Could you check a few things on this model? Use its own coordinates, in mm. Face numbers are marked on the shaded views. A direction names the side the tool comes from. Round coordinates to 2 decimals unless told otherwise and drop trailing zeros. Loops run counter-clockwise (first coordinate to the right, second up) from the corner with the lowest first, then second, coordinate; pieces in that order, holes last. Notation, with made-up numbers: M -2.5,-24.75 L 32.5,-24.75 A27 cw 32.5,-2.75 Z; hole C 21,59.5 d10. An arc over 180 degrees is marked long. Answer in a Markdown table with one row per item.
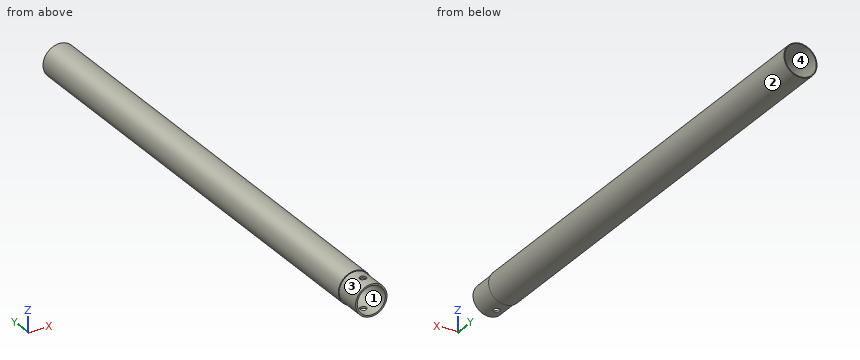
```python
from build123d import *

# Parameters (mm, degrees)
SKETCH1_R                = 31.75
SKETCH1_R_2              = 30.1625
BOSS_EXTRUDE1_DEPTH      = 914.4
BOSS_EXTRUDE2_DEPTH      = 50.8
BOSS_EXTRUDE2_DEPTH_BACK = 25.4
SKETCH3_R                = 30.1625
SKETCH3_R_2              = 26.9875
CUT_EXTRUDE2_DEPTH       = 916.501766792
CUT_EXTRUDE2_DEPTH_BACK  = 916.501766792
SKETCH7_R                = 6.35


with BuildPart() as part:
    # Sketch1 → Boss-Extrude1 (new body)
    with BuildSketch(Plane(origin=(0, 0, 0), x_dir=(1, 0, 0), z_dir=(0, 1, 0))):
        with Locations(Location((0, 0, 0), (0, 0, 270))):
            Circle(SKETCH1_R)
        with Locations(Location((0, 0, 0), (0, 0, 270))):
            Circle(SKETCH1_R_2, mode=Mode.SUBTRACT)
    extrude(amount=BOSS_EXTRUDE1_DEPTH)

    # Sketch3 → Boss-Extrude2 (add, two sides: drawn at the far end of the back side and taken through both)
    with BuildSketch(Plane.XZ.offset(-BOSS_EXTRUDE2_DEPTH_BACK)):
        with Locations(Location((0, 0, 0), (0, 0, 270))):
            Circle(SKETCH3_R)
        with Locations(Location((0, 0, 0), (0, 0, 270))):
            Circle(SKETCH3_R_2, mode=Mode.SUBTRACT)
    extrude(amount=BOSS_EXTRUDE2_DEPTH + BOSS_EXTRUDE2_DEPTH_BACK)

    # Sketch7 → Cut-Extrude2 (cut, two sides: drawn at the far end of the back side and taken through both)
    with BuildSketch(Plane.XY.offset(-CUT_EXTRUDE2_DEPTH_BACK)):
        with Locations((0, -25.4)):
            Circle(SKETCH7_R)
    extrude(amount=CUT_EXTRUDE2_DEPTH + CUT_EXTRUDE2_DEPTH_BACK, mode=Mode.SUBTRACT)


solid = part.part
```
1) I want a section at A-A, the plane z = 0. Please give me the cut outline in (x, y).
Computed:
| item | result |
|---|---|
| outline | M -31.75,0 L -30.16,0 L -30.16,-50.8 L -26.99,-50.8 L -26.99,25.4 L -30.16,25.4 L -30.16,914.4 L -31.75,914.4 Z; M 26.99,-50.8 L 30.16,-50.8 L 30.16,0 L 31.75,0 L 31.75,914.4 L 30.16,914.4 L 30.16,25.4 L 26.99,25.4 Z |
2) I need wall thicknesses on line 1 (X direction, y = -23, z = 0); line 2 (X direction, y = 825.5, z = -1); line 3 (Z direction, x = 2, y = 257.5). Which ranges of each line are inside material? Lowest first, please.
Computed:
| item | result |
|---|---|
| line 1 | x = -30.16 to -26.99, 26.99 to 30.16 |
| line 2 | x = -31.73 to -30.15, 30.15 to 31.73 |
| line 3 | z = -31.69 to -30.1, 30.1 to 31.69 |
3) Which directions (+Z, -Z, +X, -X, +Y, -Y) give clear straight access to the entire face, cutting with the end or side of a thin tool? Please do the marked faces 3 and 4.
Computed:
| item | result |
|---|---|
| face 3 | -Y |
| face 4 | +Y |
4) Will these pins go through, and if not, where does the flat tip stop? P1, Ø10, axis at x = 22, y = 526, coming from the -Z side; P2, Ø8, axis at y = 776.5, z = 3.5, coming from the +X side; P3, Ø10, axis at y = 323.5, z = 2, coming from the -X side.
Computed:
| item | result |
|---|---|
| P1 | stops at z = -26.82 |
| P2 | stops at x = 31.75 |
| P3 | stops at x = -31.75 |
5) If we mould it in two halves opening along X, with no side actions, what happens to the marked faces 1 and 2? For each: released by +X, released by -X, zero draft, split by the parting line, or undercut.
Computed:
| item | result |
|---|---|
| face 1 | undercut |
| face 2 | split by the parting line |
